Autodesk Inventor part; units mm, degrees
ref_plane "YZ Plane" through (0, 0, 0) normal (1, 0, 0) x (0, 1, 0)
ref_plane "XZ Plane" through (0, 0, 0) normal (0, 1, 0) x (-1, 0, 0)
ref_plane "XY Plane" through (0, 0, 0) normal (0, 0, 1) x (1, 0, 0)
sketch "Sketch1" plane through (0, 0, 0) normal (0, 1, 0) x (-1, 0, 0)
  line L0 (12.7, 21.75) -> (-12.7, 21.75)
  line L1 (-12.7, 21.75) -> (-12.7, -21.75)
  line L2 (-12.7, -21.75) -> (12.7, -21.75)
  line L3 (12.7, -21.75) -> (12.7, 21.75)
  line L4 (12.7, 21.75) -> (-12.7, -21.75) construction
  line L5 (-12.7, 21.75) -> (12.7, -21.75) construction
  point P0 (0, 0)
  dimension "d0" = 25.4
  dimension "d1" = 43.5
extrude "Extrusion1" add sketch "Sketch1" along normal blind 5
sketch "Sketch2" plane through (0, 5, 0) normal (0, 1, 0) x (1, 0, 0)
  point P0 (0, 0)
  point P1 (0, 0)
  dimension "d11" = 0
  dimension "d12" = 0
hole "Hole1" at (0, 5, 0) direction (0, -1, 0) diameter 6.756 depth 25.4
properties part number "stage_shim"
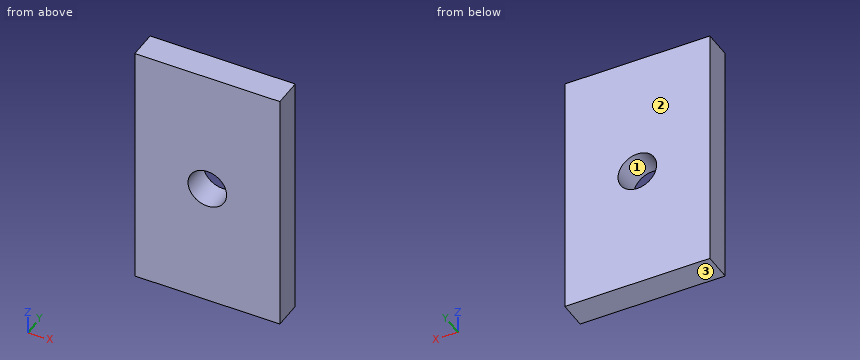
Design review of the part built by this model. Coordinates are the model's own, in mm. Face numbers are marked on the shaded views. Give positions to 0.01 mm unless a question says otherwise; leave off trailing zeros. Loops run counter-clockwise (first coordinate to the right, second up) from the corner with the lowest first, then second, coordinate; pieces in that order, holes last. Notation, with made-up numbers: M 45,49.5 L 80,49.5 A36 cw 80,85.5 Z; hole C 40.25,47 d5. An arc over 180 degrees is marked long. Answer as a JSON object with one key per item and string values.
Item 1: We need section A-A (z = 0). State the section outline as (x, y) points.
Output values:
{"outline": "M -12.7,0 L -3.38,0 L -3.38,5 L -12.7,5 Z; M 3.38,0 L 12.7,0 L 12.7,5 L 3.38,5 Z"}
Item 2: Wall thickness on line 1 along X through (y, z) = (1.05, 0); line 2 along Z through (x, y) = (0, 1.8); line 3 along Z through (x, y) = (2.5, 2.4): over which ranges is each line inside the solid? List them lowest first.
Output values:
{"line 1": "x = -12.7 to -3.38, 3.38 to 12.7", "line 2": "z = -21.75 to -3.38, 3.38 to 21.75", "line 3": "z = -21.75 to -2.27, 2.27 to 21.75"}
Item 3: We need section C-C (y = 2.4). State the section outline as (x, z) points.
Output values:
{"outline": "M -12.7,-21.75 L 12.7,-21.75 L 12.7,21.75 L -12.7,21.75 Z; hole C 0,0 d6.76"}
Item 4: Mouldability with a two-part tool opening along Z and no side actions: class the marked faces 1, 2 and 3 as pulls with the +Z half, pulls with the -Z half, needs draft (parallel to the pull), parting line crosses it, or undercut.
Output values:
{"face 1": "undercut", "face 2": "needs draft", "face 3": "pulls with the -Z half"}
Item 5: We need section B-B (x = 0). State the section outline as (y, z) points, and give its area (3 significant figures).
Output values:
{"outline": "M 0,-21.75 L 5,-21.75 L 5,-3.38 L 0,-3.38 Z; M 0,3.38 L 5,3.38 L 5,21.75 L 0,21.75 Z", "area": "184 mm2"}
